Source: CAD feature listing. Evaluate the final solid. Frame: model axes, mm. A direction names the side the tool comes from. Give positions to 0.01 mm unless a question says otherwise; leave off trailing zeros. Loops run counter-clockwise (first coordinate to the right, second up) from the corner with the lowest first, then second, coordinate; pieces in that order, holes last. Notation, with made-up numbers: (-2.5, -27.5) -> (32.5, -27.5) arc R27 cw to (32.5, -3.5) -> close; hole circle Ø4 at (53, 30.5). An arc over 180 degrees is marked (long way). Return JSON: item names as keys, results as strings. Group by question number.
```python
from build123d import *

# Parameters (mm, degrees)
SKETCH1_W           = 30
SKETCH1_H           = 20
BOSS_EXTRUDE1_DEPTH = 15
SKETCH2_W           = 5
SKETCH2_H           = 15
CUT_EXTRUDE4_DEPTH  = 17
SKETCH3_W           = 20
SKETCH3_H           = 2
CUT_EXTRUDE5_DEPTH  = 17
BOSS_EXTRUDE3_DEPTH = 4
BOSS_EXTRUDE4_DEPTH = 4
SKETCH8_R           = 1.579197179
SKETCH8_R_2         = 1.58
CUT_EXTRUDE8_DEPTH  = 4
CUT_EXTRUDE12_DEPTH = 4
SKETCH10_R          = 0.75
BOSS_EXTRUDE5_DEPTH = 3


with BuildPart() as part:
    # Sketch1 → Boss-Extrude1 (new body)
    with BuildSketch(Plane(origin=(0, 0, 0), x_dir=(1, 0, 0), z_dir=(0, 1, 0))):
        with Locations((15, 10)):
            Rectangle(SKETCH1_W, SKETCH1_H)
    extrude(amount=BOSS_EXTRUDE1_DEPTH)

    # Sketch2 → Cut-Extrude4 (cut)
    with BuildSketch(Plane.XY):
        with Locations((27.5, 7.5)):
            Rectangle(SKETCH2_W, SKETCH2_H)
        with Locations((2.5, 7.5)):
            Rectangle(SKETCH2_W, SKETCH2_H)
    extrude(amount=-CUT_EXTRUDE4_DEPTH, mode=Mode.SUBTRACT)

    # Sketch3 → Cut-Extrude5 (cut)
    with BuildSketch(Plane.XY):
        with Locations((15, 14)):
            Rectangle(SKETCH3_W, SKETCH3_H)
    extrude(amount=-CUT_EXTRUDE5_DEPTH, mode=Mode.SUBTRACT)

    # Sketch6 → Boss-Extrude3 (add)
    with BuildSketch(Plane(origin=(0, 0, -20), x_dir=(-1, 0, 0), z_dir=(0, 0, -1))):
        with BuildLine():
            Line((-8.569503225, 11.796579234), (-21.490222751, 11.796579234))
            ThreePointArc((-21.490222751, 11.796579234), (-22.407058542, 11.036037401), (-22.599660768, 9.860488113))
            Line((-22.599660768, 9.860488113), (-21.315495161, 3.650100945))
            ThreePointArc((-21.315495161, 3.650100945), (-20.823120618, 3.032864625), (-20.069739851, 2.796579234))
            Line((-20.069739851, 2.796579234), (-10.84314976, 2.796579234))
            ThreePointArc((-10.84314976, 2.796579234), (-10.281938841, 3.044467569), (-9.88839036, 3.515132967))
            Line((-9.88839036, 3.515132967), (-7.531107534, 10.273814665))
            ThreePointArc((-7.531107534, 10.273814665), (-7.826028971, 11.188134351), (-8.569503225, 11.796579234))
        make_face()
    extrude(amount=BOSS_EXTRUDE3_DEPTH)

    # Sketch7 → Boss-Extrude4 (add)
    with BuildSketch(Plane(origin=(0, 0, -20), x_dir=(-1, 0, 0), z_dir=(0, 0, -1))):
        Polygon((-3.985927745, 10.00319824), (-6.12825709, 8.766323815), (-6.12825709, 6.292574967), (-3.985927745, 5.055700542), (-1.843598399, 6.292574967), (-1.843598399, 8.766323815), align=None)
        Polygon((-25.896274691, 10.00319824), (-28.038604037, 8.766323815), (-28.038604037, 6.292574967), (-25.896274691, 5.055700542), (-23.753945346, 6.292574967), (-23.753945346, 8.766323815), align=None)
    extrude(amount=BOSS_EXTRUDE4_DEPTH)

    # Sketch8 → Cut-Extrude8 (cut)
    with BuildSketch(Plane(origin=(0, 0, -24), x_dir=(-1, 0, 0), z_dir=(0, 0, -1))):
        with Locations((-25.949762311, 7.480091341)):
            Circle(SKETCH8_R)
        with Locations((-4.010420372, 7.480091341)):
            Circle(SKETCH8_R_2)
    extrude(amount=-CUT_EXTRUDE8_DEPTH, mode=Mode.SUBTRACT)

    # Sketch9 → Cut-Extrude12 (cut)
    with BuildSketch(Plane(origin=(0, 0, -24), x_dir=(-1, 0, 0), z_dir=(0, 0, -1))):
        Polygon((-8.748681153, 10.506207471), (-21.331387013, 10.48502632), (-20.043360928, 3.411896064), (-11.018349356, 3.427088355), align=None)
    extrude(amount=-CUT_EXTRUDE12_DEPTH, mode=Mode.SUBTRACT)

    # Sketch10 → Boss-Extrude5 (add)
    with BuildSketch(Plane(origin=(0, 0, -20), x_dir=(-1, 0, 0), z_dir=(0, 0, -1))):
        with Locations(Location((-10.699729711, 9.112601358, 0), (0, 0, 180))):
            Circle(SKETCH10_R)
        with Locations(Location((-11.814614601, 6.843014261, 0), (0, 0, 180))):
            Circle(SKETCH10_R)
        with Locations(Location((-12.699729711, 9.112601358, 0), (0, 0, 180))):
            Circle(SKETCH10_R)
        with Locations(Location((-13.814614601, 6.843014261, 0), (0, 0, 180))):
            Circle(SKETCH10_R)
        with Locations(Location((-14.699729711, 9.112601358, 0), (0, 0, 180))):
            Circle(SKETCH10_R)
        with Locations(Location((-15.814614601, 6.843014261, 0), (0, 0, 180))):
            Circle(SKETCH10_R)
        with Locations(Location((-16.699729711, 9.112601358, 0), (0, 0, 180))):
            Circle(SKETCH10_R)
        with Locations(Location((-17.814614601, 6.843014261, 0), (0, 0, 180))):
            Circle(SKETCH10_R)
        with Locations(Location((-18.699729711, 9.112601358, 0), (0, 0, 180))):
            Circle(SKETCH10_R)
        with Locations(Location((-19.814614601, 6.843014261, 0), (0, 0, 180))):
            Circle(SKETCH10_R)
    extrude(amount=BOSS_EXTRUDE5_DEPTH)


solid = part.part
```
1) Cut plane A-A on x = 23. Return loops of the section in (y, z), then the cut area to 3 significant figures.
2) Contact query for flat-ended pins moving along their axis: P1, Ø0.7, axis at y = 8, z = -22.5, coming from the -X side; P2, Ø1.6, axis at x = 18.5, y = 9, coming from the -Z side; P3, Ø1, axis at y = 12.5, z = -9.5, coming from the -X side. Output: stop coordinate, or through.
3) Mould query, pull axis Y, two halves, no side actions, for faces 1 (the face through (12, 7, -23)), 2 (the face through (16, 7, -23)), 3 (the face through (24.81, 9.376, -21.972)), 4 (the face through (30, 7, -18)). Classes: released by +Y, released by -Y, zero draft, split by the parting line, or undercut.
4) Cut plane B-B on y = 2. Return loops of the section in (x, z).
5) Cut plane C-C on z = -21.25. Count the separate pieces of the cut face and the enclosed holes in it, then the cut area to 3 significant figures.
6) Cut plane D-D on z = -7. Return loops of the section in (x, y), then the cut area to 3 significant figures.
7) Material intervals for line 1 (Y direction, x = 16.75, z = -22.5); line 2 (Y direction, x = 8, z = -16.5); line 3 (Z direction, x = 28, y = 1), sorted ascending.
8) Reachability of faces 5 (the face through (15.393, 9.4, -21.479)), 6 (the face through (5.042, 9.393, -21.972)), 7 (the face through (1.844, 8, -22)) from +Z, -Z, +X, -X, +Y, -Y: full face, straight path, thin tool, end or side. Return the list, or none.
Calculated:
{
 "1": {"outline": "(0, -20) -> (15, -20) -> (15, -17) -> (13, -17) -> (13, 0) -> (0, 0) -> close", "area": "266 mm2"},
 "2": {"P1": "x = 1.84", "P2": "z = -23", "P3": "x = 5"},
 "3": {"face 1": "undercut", "face 2": "undercut", "face 3": "released by +Y", "face 4": "zero draft"},
 "4": {"outline": "(0, -20) -> (30, -20) -> (30, -17) -> (25, -17) -> (25, 0) -> (5, 0) -> (5, -17) -> (0, -17) -> close"},
 "5": {"separate pieces": "13", "enclosed holes": "3", "area": "76.8 mm2"},
 "6": {"outline": "(5, 0) -> (25, 0) -> (25, 13) -> (5, 13) -> close", "area": "260 mm2"},
 "7": {"line 1": "2.8 to 3.42, 8.36 to 9.86, 10.49 to 11.8", "line 2": "0 to 13", "line 3": "-20 to -17"},
 "8": {"face 5": "-Z", "face 6": "-Z, +Y", "face 7": "-Z, -X, +Y, -Y"}
}
